Verification items for the finished model (mm, model axes). Round coordinates to 2 decimals unless told otherwise and drop trailing zeros. Write each loop counter-clockwise with the first axis right and the second up, starting at its lowest first coordinate (ties: lowest second). Pieces come first, ordered by that corner, then holes. Notation, with made-up numbers: (64.5, 84.25) - (117.5, 84.25) arc R12 ccw to (117.5, 102.25) - close; hole circle Ø8 at (67, 23.5). An arc over 180 degrees is marked (long way). Write each question's results on one line, items separated by ' | '.
```python
from build123d import *

# Parameters (mm, degrees)
BOSS_EXTRUDE2_DEPTH     = 203.2
SKETCH4_R               = 12.7
SKETCH4_R_2             = 5.08
CUT_EXTRUDE1_DEPTH      = 76.2
CUT_EXTRUDE1_DEPTH_BACK = 92.964


with BuildPart() as part:
    # Sketch1 → Boss-Extrude2 (new body)
    with BuildSketch(Plane(origin=(0, 0, 0), x_dir=(1, 0, 0), z_dir=(0, 1, 0))):
        with BuildLine():
            Line((-6.35, -19.05), (6.35, -19.05))
            ThreePointArc((6.35, -19.05), (15.330256121, -15.330256121), (19.05, -6.35))
            Line((19.05, -6.35), (19.05, 6.35))
            ThreePointArc((19.05, 6.35), (15.330256121, 15.330256121), (6.35, 19.05))
            Line((6.35, 19.05), (-6.35, 19.05))
            ThreePointArc((-6.35, 19.05), (-15.330256121, 15.330256121), (-19.05, 6.35))
            Line((-19.05, 6.35), (-19.05, -6.35))
            ThreePointArc((-19.05, -6.35), (-15.330256121, -15.330256121), (-6.35, -19.05))
        make_face()
    extrude(amount=BOSS_EXTRUDE2_DEPTH)

    # Sketch4 → Cut-Extrude1 (cut, two sides)
    with BuildSketch(Plane.XY) as cut_extrude1_sk:
        with Locations((0, 164.846)):
            Circle(SKETCH4_R)
        with Locations((0, 6.35)):
            Circle(SKETCH4_R_2)
    extrude(amount=CUT_EXTRUDE1_DEPTH, mode=Mode.SUBTRACT)
    extrude(cut_extrude1_sk.sketch, amount=-CUT_EXTRUDE1_DEPTH_BACK, mode=Mode.SUBTRACT)


solid = part.part
```
(1) Section check D-D (z = -13.5). Record the cut outline in (x, y), plus the area to 3 significant figures.
Answer:
outline: (-16.85, 0) - (16.85, 0) - (16.85, 203.2) - (-16.85, 203.2) - close; hole circle Ø25.4 at (0, 164.85); hole circle Ø10.16 at (0, 6.35) | area: 6,260 mm2
(2) Go/stop test with flat-tipped pins: pin 1 Ø1 at (y, z) = (129, -7) entering from -X; pin 2 Ø5 at (y, z) = (175, -11.5) entering from +X. Record where each tip stops, or that it passes through.
Answer:
pin 1: x = -19.05 | pin 2: x = 18.77
(3) Section check A-A (x = 0). Record the cut outline in (y, z).
Answer:
outline: (0, -19.05) - (1.27, -19.05) - (1.27, 19.05) - (0, 19.05) - close; (11.43, -19.05) - (152.15, -19.05) - (152.15, 19.05) - (11.43, 19.05) - close; (177.55, -19.05) - (203.2, -19.05) - (203.2, 19.05) - (177.55, 19.05) - close
(4) Section check C-C (y = 148). Record the cut outline in (x, z), plus the area to 3 significant figures.
Answer:
outline: (-19.05, -6.35) arc R12.7 ccw to (-6.35, -19.05) - (6.35, -19.05) arc R12.7 ccw to (19.05, -6.35) - (19.05, 6.35) arc R12.7 ccw to (6.35, 19.05) - (-6.35, 19.05) arc R12.7 ccw to (-19.05, 6.35) - close | area: 1,310 mm2
(5) Thickness scan on L1, parallel to Y at x = 0, z = -6.75; L2, parallel to Y at x = -3.5, z = 15; L3, parallel to X at y = 176.5, z = 3.5. Record the ranges inside material, lowest first.
Answer:
L1: 0 to 1.27, 11.43 to 152.15, 177.55 to 203.2 | L2: 0 to 2.67, 10.03 to 152.64, 177.05 to 203.2 | L3: -19.05 to -5.05, 5.05 to 19.05
(6) Section check B-B (y = 6.35). Record the cut outline in (x, z).
Answer:
outline: (-19.05, -6.35) arc R12.7 ccw to (-6.35, -19.05) - (-5.08, -19.05) - (-5.08, 19.05) - (-6.35, 19.05) arc R12.7 ccw to (-19.05, 6.35) - close; (5.08, -19.05) - (6.35, -19.05) arc R12.7 ccw to (19.05, -6.35) - (19.05, 6.35) arc R12.7 ccw to (6.35, 19.05) - (5.08, 19.05) - close
